```python
from build123d import *

# Parameters (mm, degrees)
EXTRUDE_THIN1_DEPTH = 178.59375
FILLET1_R           = 1.016


with BuildPart() as part:
    # Sketch1 → Extrude-Thin1 (new body)
    with BuildSketch(Plane.XY):
        with BuildLine():
            Line((0, 17.859375), (-3.175, 17.859375))
            Line((-3.175, 17.859375), (-3.175, 15.478125))
            ThreePointArc((-3.175, 15.478125), (-5.84807115, 14.657210579), (-7.599625174, 12.477470145))
            ThreePointArc((-7.599625174, 12.477470145), (-9.638294165, 10.117590004), (-12.7, 9.525))
            Line((-12.7, 9.525), (-12.7, 6.35))
            Line((-12.7, 6.35), (-1.359217172, 6.35))
            Line((-1.359217172, 6.35), (-1.014506285, 0))
            Line((-1.014506285, 0), (0, 0.055072655))
            Line((0, 0.055072655), (-0.396875, 7.366))
            Line((-0.396875, 7.366), (-11.684, 7.366))
            Line((-11.684, 7.366), (-11.684, 8.47084132))
            ThreePointArc((-11.684, 8.47084132), (-8.641469435, 9.554461447), (-6.655705137, 12.101609848))
            ThreePointArc((-6.655705137, 12.101609848), (-4.833592242, 14.074990123), (-2.159, 14.3217318))
            Line((-2.159, 14.3217318), (-2.159, 16.843375))
            Line((-2.159, 16.843375), (0, 16.843375))
            Line((0, 16.843375), (0, 17.859375))
        make_face()
    extrude(amount=-EXTRUDE_THIN1_DEPTH)

    # Fillet1
    fillet1_edges = [part.edges().sort_by_distance(p)[0] for p in [
        (-12.7, 6.35, -89.296875),
        (-12.7, 9.525, -89.296875),
        (-3.175, 17.859375, -89.296875),
        (-2.159, 14.3217318, -89.296875),
        (-0.396875, 7.366, -89.296875),
    ]]
    fillet(fillet1_edges, radius=FILLET1_R)


solid = part.part
```
The listing builds one solid part. Answer for the finished solid, in the listing's coordinates (mm). A direction names the side the tool comes from. Give positions to 0.01 mm unless a question says otherwise; leave off trailing zeros. Write each loop counter-clockwise with the first axis right and the second up, starting at its lowest first coordinate (ties: lowest second). Pieces come first, ordered by that corner, then holes. Notation, with made-up numbers: (-15, 30.5) -> (32, 30.5) arc R20 ccw to (32, 57.5) -> close; hole circle Ø11 at (5, 76.25). An arc over 180 degrees is marked (long way). Write item = value, one per line. Start each with the question number.
1) The part is cut by section B-B, the plane y = 3. Determine the outline of the cut face in (x, z), and give its area (3 significant figures).
2) Determine the mould class of faces 1 (the face through (-7, 6.35, -88)), 2 (the face through (-5, 7, 0)), 3 (the face through (-5.3, 13.8, -88)) for opening direction Y: +Y half, -Y half, draft (parallel to the pull), parting line (faces both ways), or undercut.
3) Straight lines are drawn through the part: line 1 along Y through (x, z) = (-3.5, -85); line 2 along Y through (x, z) = (-1.5, -126.5); line 3 along X through (y, z) = (15.75, -34) (3 decimals). For each, find the intervals that lie inside material, in ascending order.
4) Each of these flat-tipped pins is pushed along its axis until it touches: pin 1 (3 mm diameter, centred on x = -8, z = -69, fed in from -Y); pin 2 (2 mm diameter, centred on y = 2, z = -84.5, fed in from -X); pin 3 (4 mm diameter, centred on x = -9.5, z = -65, fed in from +Y). Where does it stop, or does it pass through?
5) Which of the six approach directions +Z, -Z, +X, -X, +Y, -Y give full straight-line access (tool end or side, diameter ignored) to faces 4 (the face through (-6, 7.366, -88)), 5 (the face through (-5, 7, -178.594))?
Solutions:
q1.outline = (-1.18, -178.59) -> (-0.16, -178.59) -> (-0.16, 0) -> (-1.18, 0) -> close
q1.area = 182 mm²
q2.face_1 = -Y half
q2.face_2 = draft
q2.face_3 = undercut
q3.line_1 = 6.35 to 7.37, 14.45 to 15.47
q3.line_2 = 6.35 to 7.37, 16.84 to 17.86
q3.line_3 = -3.175 to -2.159
q4.pin_1 = 6.35
q4.pin_2 = -1.18
q4.pin_3 = 12.71
q5.face_4 = +Z, -Z, +X
q5.face_5 = -Z, +X, -X, +Y, -Y
